Check sheet for the modelled part. Datum: model origin and axes. Units: mm. A direction names the side the tool comes from. Coordinates: 2 decimals unless noted, no trailing zeros. Order: outer loops, then holes, each group sorted by start corner. A loop starts at its lowest first (then second) coordinate and runs counter-clockwise, first axis right, second up.
from build123d import *

# Parameters (mm, degrees)
SKETCH_1_R      = 1.6
SKETCH_1_R_2    = 1.817226884
SKETCH_1_W      = 24
SKETCH_1_H      = 34
EXTRUDE_1_DEPTH = 3


with BuildPart() as part:
    # 草图1 → 凸台-拉伸1 (new body)
    # profile 1 of 3: a face of its own
    with BuildSketch(Plane(origin=(0, 0, 0), x_dir=(1, 0, 0), z_dir=(0, 1, 0))):
        with BuildLine():
            Line((19, -17), (19, 17))
            Line((19, 17), (40, 17))
            ThreePointArc((40, 17), (42.828427126, 18.171572876), (44, 21.000000002))
            ThreePointArc((44, 21.000000002), (42.828427124, 23.828427126), (40, 25))
            Line((40, 25), (19, 25))
            Line((19, 25), (-19, 25))
            Line((-19, 25), (-19, 17))
            Line((-19, 17), (-19, -17))
            Line((-19, -17), (-19, -25))
            Line((-19, -25), (19, -25))
            Line((19, -25), (40, -25))
            ThreePointArc((40, -25), (42.828427125, -23.828427125), (44, -21))
            ThreePointArc((44, -21), (42.828427125, -18.171572875), (40, -17))
            Line((40, -17), (19, -17))
        make_face()
        with Locations(Location((21.73, -21.615, 0), (0, 0, 270))):
            Circle(SKETCH_1_R, mode=Mode.SUBTRACT)
        with Locations(Location((39.5, -21, 0), (0, 0, 270))):
            Circle(SKETCH_1_R_2, mode=Mode.SUBTRACT)
        Rectangle(SKETCH_1_W, SKETCH_1_H, mode=Mode.SUBTRACT)
        with Locations(Location((21.73, 21.615, 0), (0, 0, 270))):
            Circle(SKETCH_1_R, mode=Mode.SUBTRACT)
        with Locations(Location((39.5, 21, 0), (0, 0, 270))):
            Circle(SKETCH_1_R_2, mode=Mode.SUBTRACT)
    # profile 2 of 3: a face of its own
    with BuildSketch(Plane(origin=(0, 0, 0), x_dir=(1, 0, 0), z_dir=(0, 1, 0))):
        with BuildLine():
            Line((-19, 17), (-19, 25))
            Line((-19, 25), (-40, 25))
            ThreePointArc((-40, 25), (-44, 21), (-40, 17))
            Line((-40, 17), (-19, 17))
        make_face()
        with Locations(Location((-39.5, 21, 0), (0, 0, 270))):
            Circle(SKETCH_1_R_2, mode=Mode.SUBTRACT)
        with Locations(Location((-21.5, 21.615, 0), (0, 0, 270))):
            Circle(SKETCH_1_R, mode=Mode.SUBTRACT)
    # profile 3 of 3: a face of its own
    with BuildSketch(Plane(origin=(0, 0, 0), x_dir=(1, 0, 0), z_dir=(0, 1, 0))):
        with BuildLine():
            Line((-40, -25), (-19, -25))
            Line((-19, -25), (-19, -17))
            Line((-19, -17), (-40, -17))
            ThreePointArc((-40, -17), (-44, -21), (-40, -25))
        make_face()
        with Locations(Location((-39.5, -21, 0), (0, 0, 270))):
            Circle(SKETCH_1_R_2, mode=Mode.SUBTRACT)
        with Locations(Location((-21.5, -21.615, 0), (0, 0, 270))):
            Circle(SKETCH_1_R, mode=Mode.SUBTRACT)
    extrude(amount=EXTRUDE_1_DEPTH)


solid = part.part
(1) Cross-section at B-B (y = 2.4). Count the separate pieces of the cut face and the enclosed holes in it, and give its area (3 significant figures).
Filled in:
separate pieces: 1
enclosed holes: 9
area: 1,780 mm2
(2) Cross-section at A-A (x = -21.5). Enter the section's corners in (y, z) (3 decimals).
Filled in:
outline: (0, -25) - (3, -25) - (3, -23.215) - (0, -23.215) - close; (0, -20.015) - (3, -20.015) - (3, -17) - (0, -17) - close; (0, 17) - (3, 17) - (3, 20.015) - (0, 20.015) - close; (0, 23.215) - (3, 23.215) - (3, 25) - (0, 25) - close
(3) Go/stop test with flat-tipped pins: P1, Ø0.9, axis at y = 1.5, z = 1, coming from the +X side; P2, Ø1.5, axis at y = 2, z = 1, coming from the -X side. Record where each tip stops, or that it passes through.
Filled in:
P1: stops at x = 19
P2: stops at x = -19
(4) Release check for a two-part mould opening along Z. For faces 1 (the flat face through (-13, 0, -2)), 2 (the flat face through (-19, 1, 0)), 3 (the cylindrical face through (-19.914, 1.479, -21.823)), 4 (the flat face through (-1, 1, 25)) record: +Z half, -Z half, draft (parallel to the pull), parting line (faces both ways), or undercut.
Filled in:
face 1: draft
face 2: undercut
face 3: undercut
face 4: +Z half
(5) Thickness scan on probe 1 along X at (y, z) = (0.6, 3); probe 2 along X at (y, z) = (0.9, 21); probe 3 along X at (y, z) = (2.6, -21.5). Record the ranges inside material, lowest first.
Filled in:
probe 1: x = -19 to -12, 12 to 19
probe 2: x = -44 to -41.32, -37.68 to -22.98, -20.02 to 20.25, 23.21 to 37.68, 41.32 to 44
probe 3: x = -43.97 to -41.25, -37.75 to -23.1, -19.9 to 20.13, 23.33 to 37.75, 41.25 to 43.97
(6) Cross-section at D-D (x = -33.5). Enter the section's corners in (y, z).
Filled in:
outline: (0, -25) - (3, -25) - (3, -17) - (0, -17) - close; (0, 17) - (3, 17) - (3, 25) - (0, 25) - close
(7) Cross-section at C-C (z = 6). Enter the section's corners in (x, y).
Filled in:
outline: (-19, 0) - (-12, 0) - (-12, 3) - (-19, 3) - close; (12, 0) - (19, 0) - (19, 3) - (12, 3) - close
(8) Tool access check on faces 5 (the flat face through (0, 1, -17)), 6 (the flat face through (-30, 1, -17)), 7 (the flat face through (19, 1, 0)). Record the directions out of +Z, -Z, +X, -X, +Y, -Y that give a thin tool (end or side, any length) a straight path to the whole face; none if there is none.
Filled in:
face 5: +Y, -Y
face 6: -X, +Y, -Y
face 7: +X, +Y, -Y
